```python
from build123d import *

# Parameters (mm, degrees)
BOSS_EXTRUDE1_DEPTH = 24
CUT_EXTRUDE1_REACH  = 5
SKETCH4_R           = 1.5
SKETCH4_R_2         = 2.05


with BuildPart() as part:
    # Sketch3 → Boss-Extrude1 (new body)
    with BuildSketch(Plane.XY):
        Polygon((-16, 0), (16, 0), (16, 17.5), (8.5, 17.5), (8.5, 3), (-8.5, 3), (-8.5, 17.5), (-16, 17.5), align=None)
    extrude(amount=BOSS_EXTRUDE1_DEPTH)

    # Sketch4 → Cut-Extrude1 (cut, up to next)
    with BuildSketch(Plane(origin=(0, 3, 0), x_dir=(1, 0, 0), z_dir=(0, 1, 0)), mode=Mode.PRIVATE) as cut_extrude1_sk1:
        with Locations((0, -5)):
            Circle(SKETCH4_R)
    cut_extrude1_tool1 = extrude(cut_extrude1_sk1.sketch, amount=-CUT_EXTRUDE1_REACH, mode=Mode.PRIVATE) & part.part
    add(cut_extrude1_tool1.solids().sort_by_distance((0, 3, 5))[0], mode=Mode.SUBTRACT)
    # Sketch4 → Cut-Extrude1 (cut, up to next)
    with BuildSketch(Plane(origin=(0, 3, 0), x_dir=(1, 0, 0), z_dir=(0, 1, 0)), mode=Mode.PRIVATE) as cut_extrude1_sk2:
        with Locations((0, -12)):
            Circle(SKETCH4_R_2)
    cut_extrude1_tool2 = extrude(cut_extrude1_sk2.sketch, amount=-CUT_EXTRUDE1_REACH, mode=Mode.PRIVATE) & part.part
    add(cut_extrude1_tool2.solids().sort_by_distance((0, 3, 12))[0], mode=Mode.SUBTRACT)
    # Sketch4 → Cut-Extrude1 (cut, up to next)
    with BuildSketch(Plane(origin=(0, 3, 0), x_dir=(1, 0, 0), z_dir=(0, 1, 0)), mode=Mode.PRIVATE) as cut_extrude1_sk3:
        with Locations((0, -19)):
            Circle(SKETCH4_R)
    cut_extrude1_tool3 = extrude(cut_extrude1_sk3.sketch, amount=-CUT_EXTRUDE1_REACH, mode=Mode.PRIVATE) & part.part
    add(cut_extrude1_tool3.solids().sort_by_distance((0, 3, 19))[0], mode=Mode.SUBTRACT)


solid = part.part
```
Model file for the job. Use its own axes, mm. A direction names the side the tool comes from. Coordinates: 2 decimals unless noted, no trailing zeros. Order: outer loops, then holes, each group sorted by start corner. A loop starts at its lowest first (then second) coordinate and runs counter-clockwise, first axis right, second up. Notation, with made-up numbers: (65, -28.75) -> (73, -28.75) arc R14 ccw to (73, -7.75) -> close; hole circle Ø3 at (74, 10). An arc over 180 degrees is marked (long way). Return JSON: item names as keys, results as strings.
Item 1: Slice it at C-C (z = 5). Write the cut outline in (x, y).
Model answer:
{"outline": "(-16, 0) -> (-1.5, 0) -> (-1.5, 3) -> (-8.5, 3) -> (-8.5, 17.5) -> (-16, 17.5) -> close; (1.5, 0) -> (16, 0) -> (16, 17.5) -> (8.5, 17.5) -> (8.5, 3) -> (1.5, 3) -> close"}
Item 2: Slice it at A-A (x = 0). Write the cut outline in (y, z).
Model answer:
{"outline": "(0, 0) -> (3, 0) -> (3, 3.5) -> (0, 3.5) -> close; (0, 6.5) -> (3, 6.5) -> (3, 9.95) -> (0, 9.95) -> close; (0, 14.05) -> (3, 14.05) -> (3, 17.5) -> (0, 17.5) -> close; (0, 20.5) -> (3, 20.5) -> (3, 24) -> (0, 24) -> close"}
Item 3: Pin check, flat tips, straight feed: P1, Ø10, axis at x = 4, y = 9, coming from the -Z side; P2, Ø1.5, axis at x = 4.5, z = 21.5, coming from the +Y side. Stop position of each tip, or through.
Model answer:
{"P1": "stops at z = 0", "P2": "stops at y = 3"}
Item 4: Wall check: line 1 along Z through (x, y) = (0, 0.85); line 2 along X through (y, z) = (0.6, 5); line 3 along X through (y, z) = (0.9, 12). Give the ranges that are in metal, low to high. Write a range as from..to.
Model answer:
{"line 1": "z = 0..3.5, 6.5..9.95, 14.05..17.5, 20.5..24", "line 2": "x = -16..-1.5, 1.5..16", "line 3": "x = -16..-2.05, 2.05..16"}
Item 5: 3-axis set-ups, long thin cutter, end or side, ignore diameter. For faces 5 (the face through (-0.195, 1.521, 3.513)), 6 (the face through (8.5, 10, 12)): which of +Z, -Z, +X, -X, +Y, -Y reach the whole face in a straight line?
Model answer:
{"face 5": "+Y, -Y", "face 6": "+Z, -Z, +Y"}
Item 6: Mould opens along X. For faces 1 (the face through (-0.444, 1.521, 14.001)), 2 (the face through (-8.5, 10, 12)), 3 (the face through (16, 9, 12)), 4 (the face through (0, 1, 0)) say: pulls with the +X half, pulls with the -X half, needs draft (parallel to the pull), parting line crosses it, or undercut.
Model answer:
{"face 1": "undercut", "face 2": "undercut", "face 3": "pulls with the +X half", "face 4": "needs draft"}
Item 7: Slice it at D-D (y = 1.5). Write the cut outline in (x, z), then the cut area to 3 significant figures.
Model answer:
{"outline": "(-16, 0) -> (16, 0) -> (16, 24) -> (-16, 24) -> close; hole circle Ø4.1 at (0, 12); hole circle Ø3 at (0, 5); hole circle Ø3 at (0, 19)", "area": "741 mm²"}
Item 8: Slice it at B-B (y = 3.5). Write the cut outline in (x, z), then the cut area to 3 significant figures.
Model answer:
{"outline": "(-16, 0) -> (-8.5, 0) -> (-8.5, 24) -> (-16, 24) -> close; (8.5, 0) -> (16, 0) -> (16, 24) -> (8.5, 24) -> close", "area": "360 mm²"}
